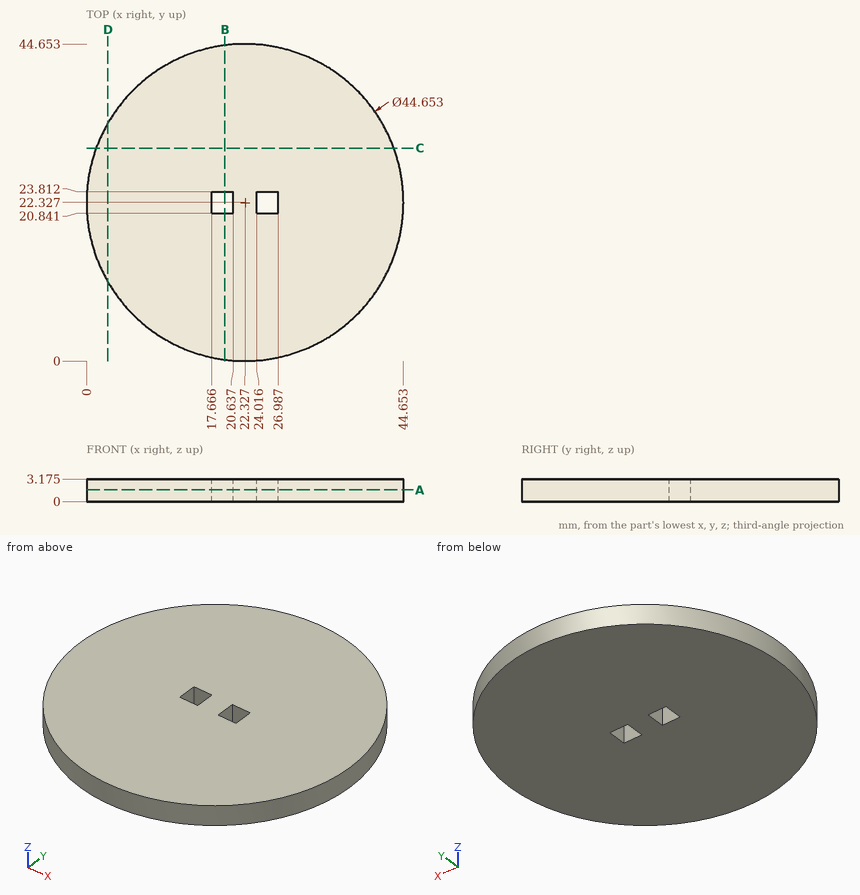
Design review of the part shown in the three views and the two pictorial views. Dimensions are in mm from the part's minimum x, y and z. Coordinates: 2 decimals unless noted, no trailing zeros. Order: outer loops, then holes, each group sorted by start corner. A loop starts at its lowest first (then second) coordinate and runs counter-clockwise, first axis right, second up.
1) Take a section at D-D, the plane x = 3. Give the boundary of the cut face in (y, z) (1 decimal).
2) Clearance check with flat-ended pins moving along their axes: pin 1 (1.5 mm diameter, centred on x = 19.5, z = 2, fed in from -Y); pin 2 (0.9 mm diameter, centred on x = 26, z = 1.5, fed in from -Y). State where each tip first meets the part, or that it passes through.
3) Take a section at B-B, the plane x = 19.5. Give the boundary of the cut face in (y, z) (1 decimal), and give its area (3 significant figures).
4) Take a section at A-A, the plane z = 1.65. Give the boundary of the cut face in (x, y) (1 decimal), and give its area (3 significant figures).
5) Wall thickness on line 1 along Y through (x, z) = (20.5, 0.25) (1 decimal); line 2 along Y through (x, z) = (16.5, 2.55) (1 decimal); line 3 along Y through (x, z) = (12, 0.95): over which ranges is each line inside the solid? List them lowest first.
6) Take a section at C-C, the plane y = 30. Give the boundary of the cut face in (x, z) (1 decimal).
Returned:
1. outline: (11.1, 0) - (33.5, 0) - (33.5, 3.2) - (11.1, 3.2) - close
2. pin 1: stops at y = 0.1
2. pin 2: stops at y = 0.23
3. outline: (0.2, 0) - (20.8, 0) - (20.8, 3.2) - (0.2, 3.2) - close; (23.8, 0) - (44.5, 0) - (44.5, 3.2) - (23.8, 3.2) - close
3. area: 131 mm2
4. outline: circle Ø44.7 at (22.3, 22.3); hole (17.7, 20.8) - (20.6, 20.8) - (20.6, 23.8) - (17.7, 23.8) - close; hole (24, 20.8) - (27, 20.8) - (27, 23.8) - (24, 23.8) - close
4. area: 1,550 mm2
5. line 1: y = 0.1 to 20.8, 23.8 to 44.6
5. line 2: y = 0.8 to 43.9
5. line 3: y = 2.53 to 42.12
6. outline: (1.4, 0) - (43.3, 0) - (43.3, 3.2) - (1.4, 3.2) - close
